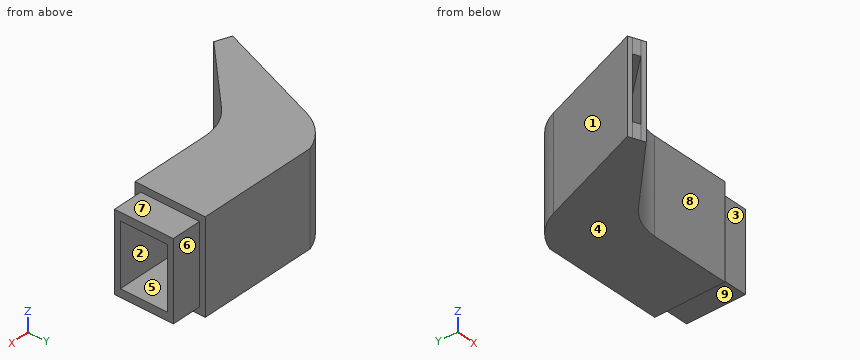
```python
from build123d import *

# Parameters (mm, degrees)
F0_W     = 17.5
F0_H     = 1.25
F1_DEPTH = 10
F0_H_2   = 10.25
F2_DEPTH = 10
F0_W_2   = 6.5
F3_DEPTH = 8.5
F4_DEPTH = 6.75
F5_DEPTH = 6.75


# Not quite as in the source:
# - a feature names something its author has since deleted; it is built from what else it names


with BuildPart() as f1:
    # F0 (on Top) → F1 (new body, symmetric)
    with BuildSketch(Plane.XY):
        with Locations((20.0137786908, 13.375)):
            Rectangle(F0_W, F0_H)
        with Locations((20.0137786908, 12.125)):
            Rectangle(F0_W, F0_H)
        with BuildLine():
            Line((2.7637786908, 11.5), (11.2637786908, 11.5))
            Line((11.2637786908, 11.5), (11.2637786908, 12.75))
            Line((11.2637786908, 12.75), (11.2637786908, 14))
            Line((11.2637786908, 14), (2.7637786908, 14))
            ThreePointArc((2.7637786908, 14), (-1.6624935941, 11.2110263052), (-4.4814392939, 6.8037816159))
            Line((-4.4814392939, 6.8037816159), (-13.0372270502, -16.686609949))
            Line((-13.0372270502, -16.686609949), (-12.1037272591, -17.0451878901))
            Line((-12.1037272591, -17.0451878901), (-3.7917014922, 5.0309925083))
            ThreePointArc((-3.7917014922, 5.0309925083), (-1.2235822128, 8.9846027287), (2.7637786908, 11.5))
        make_face()
    extrude(amount=F1_DEPTH, both=True)



with BuildPart() as f1b:
    # F0 (on Top) → F1, piece 2 (new body, symmetric)
    with BuildSketch(Plane.XY):
        with Locations((20.0137786908, 0.625)):
            Rectangle(F0_W, F0_H)
        with Locations((20.0137786908, -0.625)):
            Rectangle(F0_W, F0_H)
        with BuildLine():
            Line((11.2637786908, -1.25), (11.2637786908, 0))
            Line((11.2637786908, 0), (11.2637786908, 1.25))
            ThreePointArc((11.2637786908, 1.25), (6.1499097664, -0.1712613654), (1.9326170674, -3.3940057761))
            Line((1.9326170674, -3.3940057761), (-10.7034775723, -17.5830548019))
            Line((-10.7034775723, -17.5830548019), (-9.7699777812, -17.9416327431))
            Line((-9.7699777812, -17.9416327431), (3.6421700758, -4.483761817))
            ThreePointArc((3.6421700758, -4.483761817), (7.1371242658, -2.1224581239), (11.2637786908, -1.25))
        make_face()
    extrude(amount=F1_DEPTH, both=True)


with BuildPart() as f1_1:
    add(f1.part)

    add(f1b.part)  # F2 merges F1b
    # F0 (on Top) → F2 (join, symmetric)
    with BuildSketch(Plane.XY):
        with Locations((20.0137786908, 6.375)):
            Rectangle(F0_W, F0_H_2)
        with BuildLine():
            ThreePointArc((1.9326170674, -3.3940057761), (6.1499097664, -0.1712613654), (11.2637786908, 1.25))
            Line((11.2637786908, 1.25), (11.2637786908, 11.5))
            Line((11.2637786908, 11.5), (2.7637786908, 11.5))
            ThreePointArc((2.7637786908, 11.5), (-1.2235822128, 8.9846027287), (-3.7917014922, 5.0309925083))
            Line((-3.7917014922, 5.0309925083), (-12.1037272591, -17.0451878901))
            Line((-12.1037272591, -17.0451878901), (-10.7034775723, -17.5830548019))
            Line((-10.7034775723, -17.5830548019), (1.9326170674, -3.3940057761))
        make_face()
    extrude(amount=F2_DEPTH, both=True)

    # F0 (on Top) → F3 (join, symmetric)
    with BuildSketch(Plane.XY):
        with Locations((32.0137786908, 12.125)):
            Rectangle(F0_W_2, F0_H)
        with Locations((32.0137786908, 6.375)):
            Rectangle(F0_W_2, F0_H_2)
        with Locations((32.0137786908, 0.625)):
            Rectangle(F0_W_2, F0_H)
    extrude(amount=F3_DEPTH, both=True)

    # F0 (on Top) → F4 (cut, symmetric)
    with BuildSketch(Plane.XY):
        with Locations((20.0137786908, 6.375)):
            Rectangle(F0_W, F0_H_2)
        with BuildLine():
            ThreePointArc((1.9326170674, -3.3940057761), (6.1499097664, -0.1712613654), (11.2637786908, 1.25))
            Line((11.2637786908, 1.25), (11.2637786908, 11.5))
            Line((11.2637786908, 11.5), (2.7637786908, 11.5))
            ThreePointArc((2.7637786908, 11.5), (-1.2235822128, 8.9846027287), (-3.7917014922, 5.0309925083))
            Line((-3.7917014922, 5.0309925083), (-12.1037272591, -17.0451878901))
            Line((-12.1037272591, -17.0451878901), (-10.7034775723, -17.5830548019))
            Line((-10.7034775723, -17.5830548019), (1.9326170674, -3.3940057761))
        make_face()
    extrude(amount=F4_DEPTH, both=True, mode=Mode.SUBTRACT)

    # F0 (on Top) → F5 (cut, symmetric)
    with BuildSketch(Plane.XY):
        with Locations((32.0137786908, 6.375)):
            Rectangle(F0_W_2, F0_H_2)
    extrude(amount=F5_DEPTH, both=True, mode=Mode.SUBTRACT)


solid = f1_1.part
```
Can you work these out from the model? Positions are in its coordinate system, mm. Face numbers are marked on the shaded views. A direction names the side the tool comes from. Round coordinates to 2 decimals unless told otherwise and drop trailing zeros. Order: outer loops, then holes, each group sorted by start corner. A loop starts at its lowest first (then second) coordinate and runs counter-clockwise, first axis right, second up.
(1) I'm going to push flat-ended pins straight in: pin 1 (1 mm diameter, centred on y = 5, z = 6.5, fed in from -X); pin 2 (8.5 mm diameter, centred on x = 21.5, y = -7, fed in from -Z); pin 3 (5 mm diameter, centred on x = 23.5, z = 1, fed in from -Y); pin 4 (12 mm diameter, centred on y = 4.5, z = -1, fed in from +X). Where does each tip first touch, or does it pass through?
Results are:
pin 1: stops at x = -5.32
pin 2: passes through
pin 3: stops at y = -1.25
pin 4: stops at x = 35.26
(2) We'd pull the mould along Y, two halves only. Please class the marked faces 1, 2, 3 and 4: +Y half, -Y half, draft (parallel to the pull), parting line (faces both ways), or undercut.
Results are:
face 1: +Y half
face 2: undercut
face 3: -Y half
face 4: draft
(3) If we section it at A-A (z = -3.75): Please give me the cut outline in (x, y), plus the area to 3 significant figures.
Results are:
outline: (-13.04, -16.69) - (-12.1, -17.05) - (-3.79, 5.03) arc R11 cw to (2.76, 11.5) - (35.26, 11.5) - (35.26, 12.75) - (28.76, 12.75) - (28.76, 14) - (2.76, 14) arc R12 ccw to (-4.48, 6.8) - close; (-10.7, -17.58) - (-9.77, -17.94) - (3.64, -4.48) arc R11 cw to (11.26, -1.25) - (28.76, -1.25) - (28.76, 0) - (35.26, 0) - (35.26, 1.25) - (11.26, 1.25) arc R14 ccw to (1.93, -3.39) - close
area: 220 mm2
(4) If we section it at B-B (x = 13): Please give me the cut outline in (y, z), plus the area to 3 significant figures.
Results are:
outline: (-1.25, -10) - (14, -10) - (14, 10) - (-1.25, 10) - close; hole (1.25, -6.75) - (11.5, -6.75) - (11.5, 6.75) - (1.25, 6.75) - close
area: 167 mm2
(5) On a 3-axis mill with a long thin cutter (end or side, diameter ignored), from which of +Z, -Z, +X, -X, +Y, -Y can I reach the whole of each face in a straight line? I mean the marked faces 5, 6, 7, 8 and 9. Say none if no direction works.
Results are:
face 5: none
face 6: +Z, -Z, +X, +Y
face 7: +Z, +X, +Y, -Y
face 8: +Z, -Z, +X, -Y
face 9: -Z, +X, +Y, -Y
(6) If I drill on L1, parallel to Z at x = 2.5, y = 1; L2, parallel to Y at x = 29.5, z = 6.5; L3, parallel to Z at x = 32, y = 7, over which ranges is the centre line in solid material (lowest first)?
Results are:
L1: z = -10 to -6.75, 6.75 to 10
L2: y = 0 to 1.25, 11.5 to 12.75
L3: z = -8.5 to -6.75, 6.75 to 8.5
(7) If we section it at C-C (z = -8): Please give me the cut outline in (x, y), plus the area to 3 significant figures.
Results are:
outline: (-13.04, -16.69) - (-9.77, -17.94) - (3.64, -4.48) arc R11 cw to (11.26, -1.25) - (28.76, -1.25) - (28.76, 0) - (35.26, 0) - (35.26, 12.75) - (28.76, 12.75) - (28.76, 14) - (2.76, 14) arc R12 ccw to (-4.48, 6.8) - close
area: 734 mm2
(8) If we section it at D-D (y = 10.5): Please give me the cut outline in (x, z).
Results are:
outline: (-2.32, -10) - (28.76, -10) - (28.76, -8.5) - (35.26, -8.5) - (35.26, -6.75) - (0.7, -6.75) - (0.7, 6.75) - (35.26, 6.75) - (35.26, 8.5) - (28.76, 8.5) - (28.76, 10) - (-2.32, 10) - close
